```python
from build123d import *

# Parameters (mm, degrees)
ESQUISSE1_W        = 70
ESQUISSE1_H        = 10
BOSS_EXTRU_1_DEPTH = 5
ESQUISSE3_R        = 5
ESQUISSE3_R_2      = 2
BOSS_EXTRU_2_DEPTH = 10


with BuildPart() as part:
    # Esquisse1 → Boss.-Extru.1 (new body)
    with BuildSketch(Plane(origin=(0, 0, 0), x_dir=(1, 0, 0), z_dir=(0, 1, 0))):
        Polygon((-35, -45), (-35, -5), (-35, 5), (-35, 25), (-45, 25), (-45, -75), (-35, -75), (-35, -55), align=None)
        Rectangle(ESQUISSE1_W, ESQUISSE1_H)
        Polygon((35, 5), (35, -5), (35, -45), (35, -55), (35, -75), (45, -75), (45, 25), (35, 25), align=None)
        with Locations((0, -50)):
            Rectangle(ESQUISSE1_W, ESQUISSE1_H)
    extrude(amount=BOSS_EXTRU_1_DEPTH)

    # Esquisse3 → Boss.-Extru.2 (add)
    with BuildSketch(Plane(origin=(45, 0, 0), x_dir=(0, 0, -1), z_dir=(1, 0, 0))):
        with BuildLine():
            Line((-93.575697107, 19.005090817), (-75, 0))
            Line((-75, 0), (-75, 5))
            Line((-75, 5), (-65.90374461, 5))
            Line((-65.90374461, 5), (-86.424302893, 25.994909183))
            ThreePointArc((-86.424302893, 25.994909183), (-85.369747008, 24.386996882), (-85, 22.5))
            ThreePointArc((-85, 22.5), (-88.113003118, 17.869747008), (-93.575697107, 19.005090817))
        make_face()
        with Locations((-90, 22.5)):
            Circle(ESQUISSE3_R)
        with Locations((-90, 22.5)):
            Circle(ESQUISSE3_R_2, mode=Mode.SUBTRACT)
    extrude(amount=-BOSS_EXTRU_2_DEPTH)


solid = part.part
```
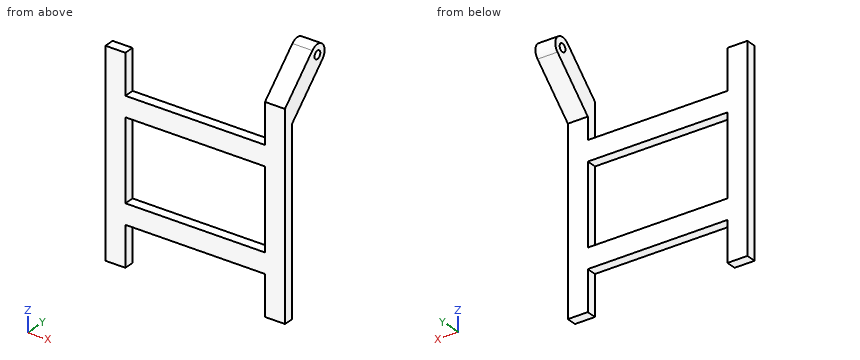
Source: CAD feature listing. Evaluate the final solid. Frame: model axes, mm. Coordinates: 2 decimals unless noted, no trailing zeros. Loops run counter-clockwise (first coordinate to the right, second up) from the corner with the lowest first, then second, coordinate; pieces in that order, holes last. Notation, with made-up numbers: (-39.75, 26) -> (-27.75, 26) arc R30 ccw to (-27.75, 54) -> close; hole circle Ø8 at (36, 13). An arc over 180 degrees is marked (long way). One line per item, written item: value. Start each with the question number.
Q1. Contact query for flat-ended pins moving along their axis: P1, Ø1.5, axis at x = -3.5, y = 3, coming from the +Z side; P2, Ø4, axis at x = 34.5, y = 18.5, coming from the -Z side; P3, Ø4.5, axis at y = 22.5, z = 90, coming from the +X side; P4, Ø3, axis at x = 35, z = 33, coming from the +Y side. Output: stop coordinate, or through.
Q2. Line query: line 1 along Z through (x, y) = (-23, 2.25); line 2 along X through (y, z) = (2.25, 59); line 3 along Y through (x, z) = (-30, -1). Output: solid intervals per line, ascending.
Q3. Section query B-B, the plane z = 7.5. Return the cut outline in (x, y).
Q4. Section query D-D, the plane z = 83. Return the cut outline in (x, y), and give its area (3 significant figures).
Q5. Section query C-C, the plane y = 12.5. Return the cut outline in (x, z).
Q6. Section query A-A, the plane x = 8. Return the cut outline in (y, z), and give its area (3 significant figures).
Results:
1. P1: z = 55
1. P2: z = 77.21
1. P3: x = 45
1. P4: y = 5
2. line 1: -5 to 5, 45 to 55
2. line 2: -45 to -35, 35 to 45
2. line 3: 0 to 5
3. outline: (-45, 0) -> (-35, 0) -> (-35, 5) -> (-45, 5) -> close; (35, 0) -> (45, 0) -> (45, 5) -> (35, 5) -> close
4. outline: (35, 8.18) -> (45, 8.18) -> (45, 22.49) -> (35, 22.49) -> close
4. area: 143 mm^2
5. outline: (35, 73.23) -> (45, 73.23) -> (45, 87.22) -> (35, 87.22) -> close
6. outline: (0, -5) -> (5, -5) -> (5, 5) -> (0, 5) -> close; (0, 45) -> (5, 45) -> (5, 55) -> (0, 55) -> close
6. area: 100 mm^2
